from build123d import *


with BuildPart() as f1:
    # F0 (on Front) → F1 (revolve)
    with BuildSketch(Plane.XZ):
        with BuildLine():
            Line((119.9262216687, -50.9453676641), (206.5908610821, -50.9453676641))
            Line((206.5908610821, -50.9453676641), (209.2918008566, -46.4251749218))
            Line((209.2918008566, -46.4251749218), (219.8045918999, -39.5420951213))
            ThreePointArc((219.8045918999, -39.5420951213), (220.5400323468, -37.6643055384), (219.0086470441, -36.3521220821))
            Line((219.0086470441, -36.3521220821), (199.2150555966, -34.5528559543))
            Line((199.2150555966, -34.5528559543), (199.2150555966, -33.0305807292))
            Line((199.2150555966, -33.0305807292), (158.9545607567, -33.0305807292))
            Line((158.9545607567, -33.0305807292), (158.9545607567, -28.323341161))
            Line((158.9545607567, -28.323341161), (135.7756108046, -28.323341161))
            Line((135.7756108046, -28.323341161), (135.7756108046, -25.0646919012))
            Line((135.7756108046, -25.0646919012), (119.9262216687, -25.0646919012))
            Line((119.9262216687, -25.0646919012), (119.9262216687, -50.9453676641))
        make_face()
    revolve(axis=Axis((113.4381368756, 0, -32.0306840586), (0, 0, -1)))

    # F2: F1 across face


with BuildPart() as f1_1:
    add(f1.part)
    add(f1.part.mirror(Plane(origin=(113.4381368756, 0, -50.9453676641), x_dir=(1, 0, 0), z_dir=(0, 0, -1))))


solid = f1_1.part
Input: part model. Units: mm. Frame: model coordinates. A direction names the side the tool comes from. Give positions to 0.01 mm unless a question says otherwise; leave off trailing zeros. Use one line per item in the form item = value.
1) First-contact query: pin 1 Ø12 at (x, y) = (177.5, -65.5) entering from +Z; pin 2 Ø1 at (x, y) = (81, -8) entering from +Z; pin 3 Ø1 at (x, y) = (48, 57) entering from +Z. Flat tips, straight axial feed; report the tip coordinate or a pass-through.
Response values:
pin_1 = -33.03
pin_2 = -28.32
pin_3 = -34.6
2) Reachability of faces 5 (the flat face through (103, 20, -28.323)), 6 (the conical face through (202.45, -28.03, -50.66)), 7 (the cylindrical face through (119.431, 2.485, -50.583)), 8 (the flat face through (150, 37, -68.86)) from +Z, -Z, +X, -X, +Y, -Y: full face, straight path, thin tool, end or side. Return the list, or none.
Response values:
face_5 = +Z
face_6 = none
face_7 = +Z, -Z
face_8 = -Z
3) Line query: probe 1 along X at (y, z) = (0, -63.5); probe 2 along Z at (x, y) = (67, 86); probe 3 along Z at (x, y) = (192, -58.5). Output: solid intervals per line, ascending.
Response values:
probe_1 = 6.31 to 106.95, 119.93 to 220.56
probe_2 = -66.25 to -56.7, -45.19 to -35.64
probe_3 = -66.23 to -56.84, -45.05 to -35.66
4) Mould query, pull axis Z, two halves, no side actions, for faces 1 (the conical face through (17.02, -4.243, -45.995)), 2 (the cylindrical face through (195.254, -25.765, -33.781)), 3 (the conical face through (202.45, -28.03, -51.23)), 4 (the conical face through (153.46, 76.95, -67.25)). Classes: pulls with the +Z half, pulls with the -Z half, needs draft (parallel to the pull), parting line crosses it, or undercut.
Response values:
face_1 = undercut
face_2 = needs draft
face_3 = undercut
face_4 = pulls with the -Z half
